The drawing under review shows one solid part. Ordinate dimensions are in mm from its lowest x, y, z. Coordinates: 2 decimals unless noted, no trailing zeros. Loops run counter-clockwise (first coordinate to the right, second up) from the corner with the lowest first, then second, coordinate; pieces in that order, holes last. Notation, with made-up numbers: M -24,37.25 L 31,37.25 A13 cw 31,58.25 Z; hole C 62,12 d9. An arc over 180 degrees is marked long. Put each result on its own line as item: value.
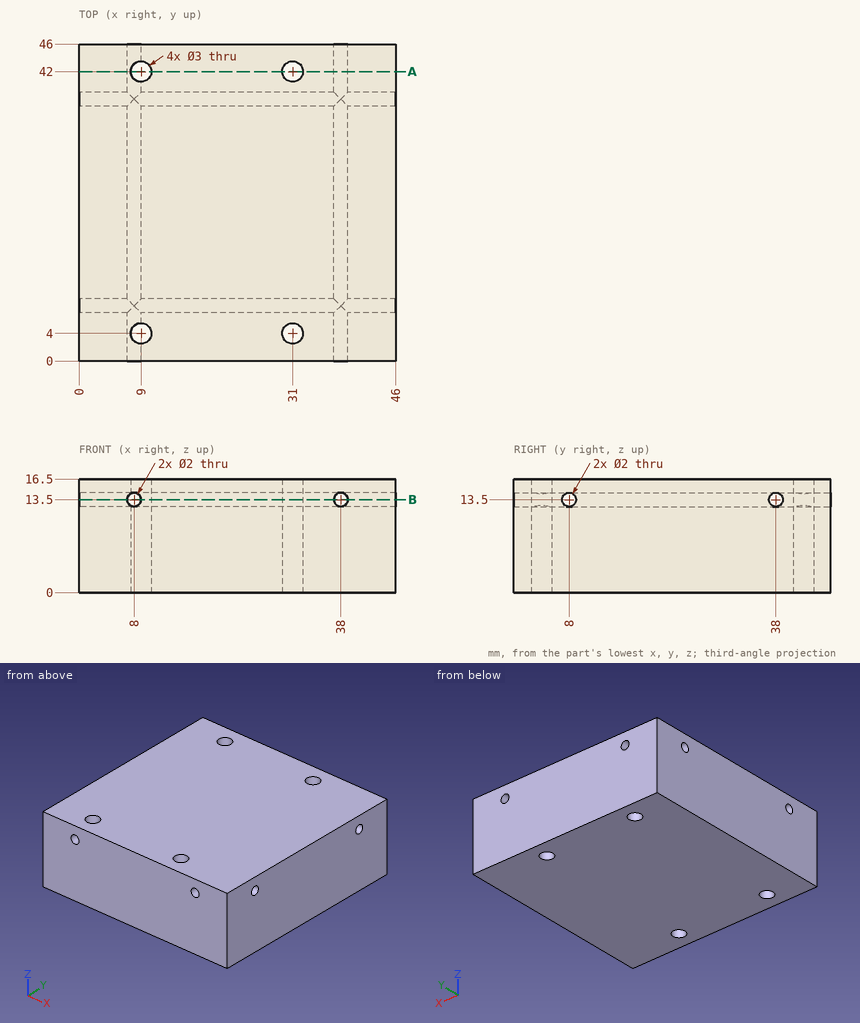
(1) Add section A-A (y = 42). Write out the cut boundary in (x, z).
Determined:
outline: M 0,0 L 7.5,0 L 7.5,12.63 A1 cw 7.5,14.37 L 7.5,16.5 L 0,16.5 Z; M 10.5,0 L 29.5,0 L 29.5,16.5 L 10.5,16.5 Z; M 32.5,0 L 46,0 L 46,16.5 L 32.5,16.5 Z; hole C 38,13.5 d2
(2) Wall thickness on line 1 along X through (y, z) = (4, 13.5); line 2 along Y through (x, z) = (9, 11); line 3 along X through (y, z) = (4, 8.5): over which ranges is each line inside the solid? List them lowest first. Write a range as [from, to].
Determined:
line 1: x = [0, 7], [10.5, 29.5], [32.5, 37], [39, 46]
line 2: y = [0, 2.5], [5.5, 40.5], [43.5, 46]
line 3: x = [0, 7.5], [10.5, 29.5], [32.5, 46]
(3) Add section B-B (z = 13.5). State how many separate pieces and enclosed holes the cut face has, plus the area to 3 significant figures.
Determined:
separate pieces: 9
enclosed holes: 2
area: 1,740 mm^2
